Geometry check sheet. Reference: the model listing, model coordinates, mm. A direction names the side the tool comes from. Round coordinates to 2 decimals unless told otherwise and drop trailing zeros. Write each loop counter-clockwise with the first axis right and the second up, starting at its lowest first coordinate (ties: lowest second). Pieces come first, ordered by that corner, then holes. Notation, with made-up numbers: (26, -29) - (81, -29) arc R18 cw to (81, -3) - close; hole circle Ø7 at (81, 47). An arc over 180 degrees is marked (long way). One line per question, with ' | ' between items. Start each with the question number.
from build123d import *

# Parameters (mm, degrees)
F0_W     = 91.952633
F0_H     = 110.787436
F1_DEPTH = 25.4
F2_R     = 12.7
F3_R     = 12.002281
F4_DEPTH = 25.4
F5_R     = 14.878246
F6_DEPTH = 12.7


with BuildPart() as f1:
    # F0 (on Top) → F1 (new body)
    with BuildSketch(Plane.XY):
        with Locations((-0.07054, 15.842587)):
            Rectangle(F0_W, F0_H)
    extrude(amount=F1_DEPTH)

    # F2
    f2_edges = [f1.edges().sort_by_distance(p)[0] for p in [
        (45.905776, -39.551131, 12.7),
    ]]
    fillet(f2_edges, radius=F2_R)

    # F3 (on face) → F4 (join)
    with BuildSketch(Plane.XY.offset(25.4)):
        with Locations((26.824998, -15.86362)):
            Circle(F3_R)
    extrude(amount=F4_DEPTH)

    # F5 (on face) → F6 (cut)
    with BuildSketch(Plane.XY.offset(25.4)):
        with Locations((-23.274958, 14.206306)):
            Circle(F5_R)
    extrude(amount=-F6_DEPTH, mode=Mode.SUBTRACT)


solid = f1.part
Q1. Draft check along Y on faces 3 (the cylindrical face through (-25.21, 28.96, 19.14)), 4 (the flat face through (-7, -39.551, 13)), 5 (the flat face through (-23, 14, 12.7)), 6 (the flat face through (45.906, 22, 13)). Enter one of: pulls with the +Y half, pulls with the -Y half, needs draft (parallel to the pull), parting line crosses it, or undercut.
Q2. Thickness scan on line 1 (Z direction, x = 30, y = 22); line 2 (Y direction, x = -22, z = 24); line 3 (Y direction, x = -20.5, z = 24). Record the ranges inside material, lowest first.
Q3. Set-up check for faces 1 (the cylindrical face through (14.834, -15.336, 37.922)), 2 (the flat face through (-1, 71.236, 13)): record each of +Z, -Z, +X, -X, +Y, -Y from which the full face is reachable in a straight line by a thin tool's end or side.
Q4. Section check A-A, the plane y = 8.5. Record the cut outline in (x, z).
Q5. Go/stop test with flat-tipped pins: P1, Ø3, axis at x = 15, z = 32, coming from the -Y side; P2, Ø6, axis at x = -8, y = -27, coming from the +Z side; P3, Ø6, axis at x = -2, y = -13.5, coming from the -Z side; P4, Ø1.5, axis at x = -22, y = 10, coming from the +Z side. Record where each tip stops, or that it passes through.
Q6. Section check D-D, the plane z = 29.5. Record the cut outline in (x, y) (3 decimals).
Q7. Section check C-C, the plane z = 21. Record the cut outline in (x, y), then the cut area to 3 significant figures.
Q8. Section check B-B, the plane x = -35.5. Record the cut outline in (y, z).
Result sheet:
1) face 3: undercut | face 4: pulls with the -Y half | face 5: undercut | face 6: needs draft
2) line 1: 0 to 25.4 | line 2: -39.55 to -0.62, 29.03 to 71.24 | line 3: -39.55 to -0.41, 28.82 to 71.24
3) face 1: +Z | face 2: +Z, -Z, +X, -X, +Y
4) outline: (-46.05, 0) - (45.91, 0) - (45.91, 25.4) - (-9.53, 25.4) - (-9.53, 12.7) - (-37.02, 12.7) - (-37.02, 25.4) - (-46.05, 25.4) - close
5) P1: y = -21.98 | P2: z = 25.4 | P3: z = 0 | P4: z = 12.7
6) outline: circle Ø24.005 at (26.825, -15.864)
7) outline: (-46.05, -39.55) - (33.21, -39.55) arc R12.7 ccw to (45.91, -26.85) - (45.91, 71.24) - (-46.05, 71.24) - close; hole circle Ø29.76 at (-23.27, 14.21) | area: 9,460 mm²
8) outline: (-39.55, 0) - (71.24, 0) - (71.24, 25.4) - (22.69, 25.4) - (22.69, 12.7) - (5.73, 12.7) - (5.73, 25.4) - (-39.55, 25.4) - close
